Work out the finished part from the listing and answer in its coordinate system (mm). Face numbers are marked on the shaded views. Coordinates: 2 decimals unless noted, no trailing zeros. Loops run counter-clockwise (first coordinate to the right, second up) from the corner with the lowest first, then second, coordinate; pieces in that order, holes last. Notation, with made-up numbers: (25.25, -20) -> (79.25, -20) arc R22 ccw to (79.25, 1) -> close; hole circle Ø7 at (79.25, -3.5). An arc over 180 degrees is marked (long way). Answer as CSV lines item,"result".
```python
from build123d import *

# Parameters (mm, degrees)
SALIENTE_EXTRUIR1_DEPTH = 12.5
REDONDEO1_R             = 2
CORTAR_EXTRUIR1_REACH   = 57.32


with BuildPart() as part:
    # Croquis1 → Saliente-Extruir1 (new body)
    with BuildSketch(Plane.XY):
        with BuildLine():
            Line((-30, 28), (30, 28))
            Line((30, 28), (30, 21))
            Line((30, 21), (15.329709717, 21))
            ThreePointArc((15.329709717, 21), (25.881503097, -2.479475236), (11.063829787, -23.528528863))
            ThreePointArc((11.063829787, -23.528528863), (7.737641456, -22.330000105), (8.936170213, -19.003811774))
            ThreePointArc((8.936170213, -19.003811774), (0, 21), (-8.936170213, -19.003811774))
            ThreePointArc((-8.936170213, -19.003811774), (-7.737641456, -22.330000105), (-11.063829787, -23.528528863))
            ThreePointArc((-11.063829787, -23.528528863), (-25.881503097, -2.479475236), (-15.329709717, 21))
            Line((-15.329709717, 21), (-30, 21))
            Line((-30, 21), (-30, 28))
        make_face()
    extrude(amount=SALIENTE_EXTRUIR1_DEPTH)

    # Redondeo1
    # the kernel refuses this fillet: 2 mm, written as the material it takes off along each edge
    with BuildSketch(Plane(origin=(0, 0, 0), x_dir=(-0.4255319148936173, -0.9049434177930525, 0), z_dir=(0.9049434177930525, -0.4255319148936173, 0))) as redondeo1_piece_1_section:
        with BuildLine():
            CenterArc((26 - REDONDEO1_R, -REDONDEO1_R), REDONDEO1_R, 0, 90)
            Line((26 - REDONDEO1_R, 0), (26, 0))
            Line((26, 0), (26, -REDONDEO1_R))
        make_face()
    redondeo1_piece_1 = revolve(axis=Axis((0, 0, 0), (0, 0, -1)), revolution_arc=129.712854224, mode=Mode.PRIVATE)
    redondeo1_piece_1 = split(redondeo1_piece_1, bisect_by=Plane(origin=(-25.427272667, 21, 0.558955185), z_dir=(0, -1, 0)), keep=Keep.TOP, mode=Mode.PRIVATE)
    add(redondeo1_piece_1, mode=Mode.SUBTRACT)
    with BuildSketch(Plane(origin=(-30, 16, 0), x_dir=(0, 0, 1), z_dir=(0, 1, 0)), Plane(origin=(30, 33, 0), x_dir=(0, 0, 1), z_dir=(0, -1, 0))) as redondeo1_piece_2:
        with BuildLine():
            CenterArc((REDONDEO1_R, REDONDEO1_R), REDONDEO1_R, 180, 90)
            Line((0, REDONDEO1_R), (0, 0))
            Line((0, 0), (REDONDEO1_R, 0))
        make_face()
    extrude(amount=17, mode=Mode.SUBTRACT)
    with BuildSketch(Plane(origin=(0, 0, 0), x_dir=(0.4242438227476812, 0.9055479992029324, 0), z_dir=(-0.9055479992029324, 0.4242438227476812, 0))) as redondeo1_piece_3_section:
        with BuildLine():
            CenterArc((26 - REDONDEO1_R, -REDONDEO1_R), REDONDEO1_R, 0, 90)
            Line((26 - REDONDEO1_R, 0), (26, 0))
            Line((26, 0), (26, -REDONDEO1_R))
        make_face()
    redondeo1_piece_3 = revolve(axis=Axis((0, 0, 0), (0, 0, -1)), revolution_arc=129.712854224, mode=Mode.PRIVATE)
    redondeo1_piece_3 = split(redondeo1_piece_3, bisect_by=Plane(origin=(25.427272718, 21, 0.558955134), z_dir=(0, -1, 0)), keep=Keep.TOP, mode=Mode.PRIVATE)
    add(redondeo1_piece_3, mode=Mode.SUBTRACT)
    with BuildSketch(Plane(origin=(10, -21.266170318, 0), x_dir=(0.42553191489361814, -0.9049434177930521, 0), z_dir=(0.9049434177930521, 0.42553191489361814, 0))) as redondeo1_piece_4:
        with BuildLine():
            CenterArc((2.5 - REDONDEO1_R, -REDONDEO1_R), REDONDEO1_R, 0, 90)
            Line((2.5 - REDONDEO1_R, 0), (2.5, 0))
            Line((2.5, 0), (2.5, -REDONDEO1_R))
        make_face()
    revolve(axis=Axis((10, -21.266170318, 0), (0, 0, -1)), revolution_arc=180, mode=Mode.SUBTRACT)
    with BuildSketch(Plane(origin=(30, 33, 12.5), x_dir=(0, 0, -1), z_dir=(0, -1, 0)), Plane(origin=(-30, 16, 12.5), x_dir=(0, 0, -1), z_dir=(0, 1, 0))) as redondeo1_piece_5:
        with BuildLine():
            CenterArc((REDONDEO1_R, -REDONDEO1_R), REDONDEO1_R, 90, 90)
            Line((0, -REDONDEO1_R), (0, 0))
            Line((0, 0), (REDONDEO1_R, 0))
        make_face()
    extrude(amount=17, mode=Mode.SUBTRACT)
    with BuildSketch(Plane(origin=(0, 0, 12.5), x_dir=(-0.4255319148936173, -0.9049434177930525, 0), z_dir=(0.9049434177930525, -0.4255319148936173, 0))) as redondeo1_piece_6_section:
        with BuildLine():
            CenterArc((26 - REDONDEO1_R, REDONDEO1_R), REDONDEO1_R, 270, 90)
            Line((26 - REDONDEO1_R, 0), (26, 0))
            Line((26, 0), (26, REDONDEO1_R))
        make_face()
    redondeo1_piece_6 = revolve(axis=Axis((0, 0, 12.5), (0, 0, -1)), revolution_arc=129.712854224, mode=Mode.PRIVATE)
    redondeo1_piece_6 = split(redondeo1_piece_6, bisect_by=Plane(origin=(-25.427272667, 21, 11.941044815), z_dir=(0, -1, 0)), keep=Keep.TOP, mode=Mode.PRIVATE)
    add(redondeo1_piece_6, mode=Mode.SUBTRACT)
    with BuildSketch(Plane(origin=(-10, -21.266170318, 12.5), x_dir=(0.42553191489361525, 0.9049434177930535, 0), z_dir=(-0.9049434177930535, 0.42553191489361525, 0))) as redondeo1_piece_7:
        with BuildLine():
            CenterArc((2.5 - REDONDEO1_R, REDONDEO1_R), REDONDEO1_R, 270, 90)
            Line((2.5 - REDONDEO1_R, 0), (2.5, 0))
            Line((2.5, 0), (2.5, REDONDEO1_R))
        make_face()
    revolve(axis=Axis((-10, -21.266170318, 12.5), (0, 0, -1)), revolution_arc=180, mode=Mode.SUBTRACT)
    with BuildSketch(Plane(origin=(0, 0, 12.5), x_dir=(0.4255319148936173, -0.9049434177930525, 0), z_dir=(-0.9049434177930525, -0.4255319148936173, 0))) as redondeo1_piece_8:
        with BuildLine():
            CenterArc((21 + REDONDEO1_R, -REDONDEO1_R), REDONDEO1_R, 90, 90)
            Line((21 + REDONDEO1_R, 0), (21, 0))
            Line((21, 0), (21, -REDONDEO1_R))
        make_face()
    revolve(axis=Axis((0, 0, 12.5), (0, 0, 1)), revolution_arc=309.631326932, mode=Mode.SUBTRACT)
    with BuildSketch(Plane(origin=(10, -21.266170318, 12.5), x_dir=(0.42553191489361814, -0.9049434177930521, 0), z_dir=(0.9049434177930521, 0.42553191489361814, 0))) as redondeo1_piece_9:
        with BuildLine():
            CenterArc((2.5 - REDONDEO1_R, REDONDEO1_R), REDONDEO1_R, 270, 90)
            Line((2.5 - REDONDEO1_R, 0), (2.5, 0))
            Line((2.5, 0), (2.5, REDONDEO1_R))
        make_face()
    revolve(axis=Axis((10, -21.266170318, 12.5), (0, 0, -1)), revolution_arc=180, mode=Mode.SUBTRACT)
    with BuildSketch(Plane(origin=(0, 0, 12.5), x_dir=(0.4242438227476812, 0.9055479992029324, 0), z_dir=(-0.9055479992029324, 0.4242438227476812, 0))) as redondeo1_piece_10_section:
        with BuildLine():
            CenterArc((26 - REDONDEO1_R, REDONDEO1_R), REDONDEO1_R, 270, 90)
            Line((26 - REDONDEO1_R, 0), (26, 0))
            Line((26, 0), (26, REDONDEO1_R))
        make_face()
    redondeo1_piece_10 = revolve(axis=Axis((0, 0, 12.5), (0, 0, -1)), revolution_arc=129.712854224, mode=Mode.PRIVATE)
    redondeo1_piece_10 = split(redondeo1_piece_10, bisect_by=Plane(origin=(25.427272718, 21, 11.941044866), z_dir=(0, -1, 0)), keep=Keep.TOP, mode=Mode.PRIVATE)
    add(redondeo1_piece_10, mode=Mode.SUBTRACT)
    with BuildSketch(Plane(origin=(0, 0, 0), x_dir=(0.4255319148936173, -0.9049434177930525, 0), z_dir=(-0.9049434177930525, -0.4255319148936173, 0))) as redondeo1_piece_11:
        with BuildLine():
            CenterArc((21 + REDONDEO1_R, REDONDEO1_R), REDONDEO1_R, 180, 90)
            Line((21 + REDONDEO1_R, 0), (21, 0))
            Line((21, 0), (21, REDONDEO1_R))
        make_face()
    revolve(axis=Axis((0, 0, 0), (0, 0, 1)), revolution_arc=309.631326932, mode=Mode.SUBTRACT)
    with BuildSketch(Plane(origin=(-10, -21.266170318, 0), x_dir=(0.42553191489361525, 0.9049434177930535, 0), z_dir=(-0.9049434177930535, 0.42553191489361525, 0))) as redondeo1_piece_12:
        with BuildLine():
            CenterArc((2.5 - REDONDEO1_R, -REDONDEO1_R), REDONDEO1_R, 0, 90)
            Line((2.5 - REDONDEO1_R, 0), (2.5, 0))
            Line((2.5, 0), (2.5, -REDONDEO1_R))
        make_face()
    revolve(axis=Axis((-10, -21.266170318, 0), (0, 0, -1)), revolution_arc=180, mode=Mode.SUBTRACT)

    # Croquis3 → Cortar-Extruir1 (cut, up to next)
    with BuildSketch(Plane.XZ.offset(-21), mode=Mode.PRIVATE) as cortar_extruir1_sk1:
        with BuildLine():
            Line((-22.25, 8.25), (-22.25, 4.25))
            ThreePointArc((-22.25, 4.25), (-24, 2.5), (-25.75, 4.25))
            Line((-25.75, 4.25), (-25.75, 8.25))
            ThreePointArc((-25.75, 8.25), (-24, 10), (-22.25, 8.25))
        make_face()
    cortar_extruir1_tool1 = extrude(cortar_extruir1_sk1.sketch, amount=-CORTAR_EXTRUIR1_REACH, mode=Mode.PRIVATE) & part.part
    # Croquis3 → Cortar-Extruir1 (cut, up to next)
    with BuildSketch(Plane.XZ.offset(-21), mode=Mode.PRIVATE) as cortar_extruir1_sk2:
        with BuildLine():
            Line((25.75, 8.25), (25.75, 4.25))
            ThreePointArc((25.75, 4.25), (24, 2.5), (22.25, 4.25))
            Line((22.25, 4.25), (22.25, 8.25))
            ThreePointArc((22.25, 8.25), (24, 10), (25.75, 8.25))
        make_face()
    cortar_extruir1_tool2 = extrude(cortar_extruir1_sk2.sketch, amount=-CORTAR_EXTRUIR1_REACH, mode=Mode.PRIVATE) & part.part
    add(cortar_extruir1_tool1.solids().sort_by_distance((-24, 21, 6.25))[0], mode=Mode.SUBTRACT)
    add(cortar_extruir1_tool2.solids().sort_by_distance((24, 21, 6.25))[0], mode=Mode.SUBTRACT)


solid = part.part
```
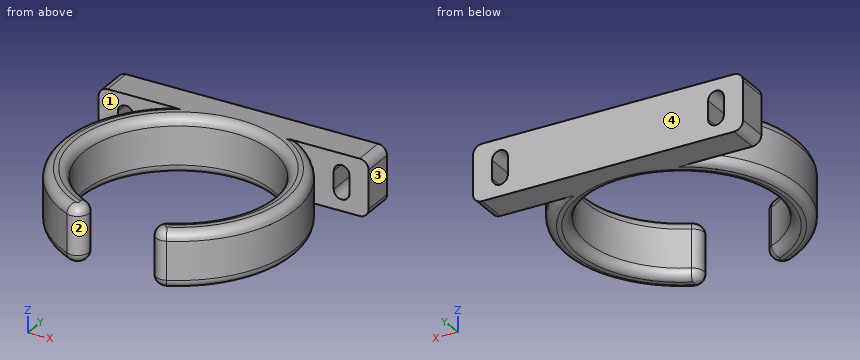
(1) A cutting plane is placed at A-A, the plane y = 0. Write down the section's boundary in (x, z).
Computed values:
outline,"(-26, 2) arc R2 ccw to (-24, 0) -> (-23, 0) arc R2 ccw to (-21, 2) -> (-21, 10.5) arc R2 ccw to (-23, 12.5) -> (-24, 12.5) arc R2 ccw to (-26, 10.5) -> close; (21, 2) arc R2 ccw to (23, 0) -> (24, 0) arc R2 ccw to (26, 2) -> (26, 10.5) arc R2 ccw to (24, 12.5) -> (23, 12.5) arc R2 ccw to (21, 10.5) -> close"
(2) Consider line 1 along X through (y, z) = (26.5, 5.75); line 2 along X through (y, z) = (0, 9.25); line 3 along Y through (x, z) = (18, 8). Determine where each line is inside the solid, lowest interval first.
Computed values:
line 1,"-30 to -25.75, -22.25 to 22.25, 25.75 to 30"
line 2,"-26 to -21, 21 to 26"
line 3,"-18.76 to -10.82, 10.82 to 18.76, 21 to 28"
(3) For a pull along Y with two mould halves and no side action, classify the marked faces 1, 2, 3 and 4 as pulls with the +Y half, pulls with the -Y half, needs draft (parallel to the pull), parting line crosses it, or undercut.
Computed values:
face 1,"undercut"
face 2,"undercut"
face 3,"needs draft"
face 4,"pulls with the +Y half"
(4) A cutting plane is placed at B-B, the plane z = 6.75. Write down the section's boundary in (x, y), and give its area (3 significant figures).
Computed values:
outline,"(-30, 21) -> (-25.75, 21) -> (-25.75, 28) -> (-30, 28) -> close; (-22.25, 21) -> (-15.33, 21) arc R26 ccw to (-11.06, -23.53) arc R2.5 ccw to (-8.94, -19) arc R21 cw (long way) to (8.94, -19) arc R2.5 ccw to (11.06, -23.53) arc R26 ccw to (15.33, 21) -> (22.25, 21) -> (22.25, 28) -> (-22.25, 28) -> close; (25.75, 21) -> (30, 21) -> (30, 28) -> (25.75, 28) -> close"
area,"921 mm2"
(5) Flat-ended cylindrical pins translate along their axes: pin 1 Ø2 at (y, z) = (-3.5, 10) entering from +X; pin 2 Ø1.5 at (y, z) = (8.5, 2) entering from +X; pin 3 Ø1 at (x, y) = (14.5, 20) entering from -Z. Find the tip coordinate at first contact, or state that the pin passes through.
Computed values:
pin 1,"x = 25.88"
pin 2,"x = 24.82"
pin 3,"z = 0.01"
